Read the model definition and answer for the solid it produces. Units are mm, in the model's axes. A direction names the side the tool comes from. Round coordinates to 2 decimals unless told otherwise and drop trailing zeros. Loops run counter-clockwise (first coordinate to the right, second up) from the corner with the lowest first, then second, coordinate; pieces in that order, holes last. Notation, with made-up numbers: (-5.5, 29) -> (36.5, 29) arc R17 ccw to (36.5, 43) -> close; hole circle Ø5 at (-29.75, 14). An arc over 180 degrees is marked (long way). Put each result on its own line as item: value.
from build123d import *

# Parameters (mm, degrees)
SKETCH_1_W         = 5.2
SKETCH_1_H         = 5.2
EXTRUDE_1_DEPTH    = 0.8
CHAMFER_1_SIZE     = 1
EXTRUDE_1_2_DEPTH  = 0.4
SKETCH_2_R         = 1
EXTRUDE_1110_DEPTH = 1.1
SKETCH_4_W         = 0.6
SKETCH_4_H         = 2.66831223
EXTRUDE_2_DEPTH    = 0.2


with BuildPart() as part:
    # 草图1 → Extrude 1 (new body)
    with BuildSketch(Plane(origin=(0, 0, 0), x_dir=(1, 0, 0), z_dir=(0, 1, 0))):
        Rectangle(SKETCH_1_W, SKETCH_1_H)
    extrude(amount=EXTRUDE_1_DEPTH)

    # 倒角1
    chamfer_1_edges = [part.edges().sort_by_distance(p)[0] for p in [
        (-2.6, 0.4, -2.6),
        (2.6, 0.4, -2.6),
        (2.6, 0.4, 2.6),
        (-2.6, 0.4, 2.6),
    ]]
    chamfer(chamfer_1_edges, length=CHAMFER_1_SIZE)

    # 草图3 → Extrude 1 2 (add)
    with BuildSketch(Plane(origin=(0, 0.8, 0), x_dir=(1, 0, 0), z_dir=(0, 1, 0))):
        Polygon((-2.1, 1.392893219), (-2.1, -1.392893219), (-1.392893219, -2.1), (1.392893219, -2.1), (2.1, -1.392893219), (2.1, 1.392893219), (1.392893219, 2.1), (-1.392893219, 2.1), align=None)
    extrude(amount=EXTRUDE_1_2_DEPTH)

    # 草图2 → Extrude 1110 (add)
    with BuildSketch(Plane(origin=(0, 1.2, 0), x_dir=(-1, 0, 0), z_dir=(0, 1, 0))):
        with Locations(Location((0, 0, 0), (0, 0, 90))):
            Circle(SKETCH_2_R)
    extrude(amount=EXTRUDE_1110_DEPTH)

    # 草图4 → 凸台-拉伸2 (add)
    with BuildSketch(Plane.XZ):
        with Locations((-1.85, 2.465843885)):
            Rectangle(SKETCH_4_W, SKETCH_4_H)
        with Locations((1.85, 2.465843885)):
            Rectangle(SKETCH_4_W, SKETCH_4_H)
        with Locations((1.85, -2.465843885)):
            Rectangle(SKETCH_4_W, SKETCH_4_H)
        with Locations((-1.85, -2.465843885)):
            Rectangle(SKETCH_4_W, SKETCH_4_H)
    extrude(amount=-EXTRUDE_2_DEPTH)


solid = part.part
Item 1: Which of the six approach directions +Z, -Z, +X, -X, +Y, -Y give full straight-line access (tool end or side, diameter ignored) to faces 1 (the flat face through (0, 2.3, 0)), 2 (the cylindrical face through (-1, 2, 0))?
Derived:
face 1: +Z, -Z, +X, -X, +Y
face 2: +Y
Item 2: The part is cut by section B-B (x = 0). Determine the outline of the cut face in (y, z), then the cut area to 3 significant figures.
Derived:
outline: (0, -2.6) -> (0.8, -2.6) -> (0.8, -2.1) -> (1.2, -2.1) -> (1.2, -1) -> (2.3, -1) -> (2.3, 1) -> (1.2, 1) -> (1.2, 2.1) -> (0.8, 2.1) -> (0.8, 2.6) -> (0, 2.6) -> close
area: 8.04 mm^2
Item 3: Flat-ended cylindrical pins translate along their axes: pin 1 Ø1 at (y, z) = (2, -2.5) entering from -X; pin 2 Ø0.5 at (x, z) = (-2, -3) entering from +Y; pin 3 Ø1 at (y, z) = (1, -3) entering from -X; pin 4 Ø0.9 at (x, y) = (-0.5, 0.5) entering from +Z. Find the tip coordinate at first contact, or state that the pin passes through.
Derived:
pin 1: passes through
pin 2: stops at y = 0.2
pin 3: stops at x = -1.66
pin 4: stops at z = 2.6
Item 4: The part is cut by section C-C (y = 1.05). Determine the outline of the cut face in (x, z), then the cut area to 3 significant figures.
Derived:
outline: (-2.1, -1.39) -> (-1.39, -2.1) -> (1.39, -2.1) -> (2.1, -1.39) -> (2.1, 1.39) -> (1.39, 2.1) -> (-1.39, 2.1) -> (-2.1, 1.39) -> close
area: 16.6 mm^2
Item 5: Find the intervals of material crossed by line 1 along Y through (x, z) = (2, 1); line 2 along Y through (x, z) = (-0.75, 2.5); line 3 along X through (y, z) = (0.9, -1), in increasing order.
Derived:
line 1: y = 0 to 1.2
line 2: y = 0 to 0.8
line 3: x = -2.1 to 2.1
Item 6: The part is cut by section D-D (z = 2.5). Determine the outline of the cut face in (x, y), then the cut area to 3 significant figures.
Derived:
outline: (-2.15, 0) -> (2.15, 0) -> (2.15, 0.2) -> (1.7, 0.2) -> (1.7, 0.8) -> (-1.7, 0.8) -> (-1.7, 0.2) -> (-2.15, 0.2) -> close
area: 2.90 mm^2
Item 7: The part is cut by section A-A (z = -3). Determine the outline of the cut face in (x, y), then the cut area to 3 significant figures.
Derived:
outline: (-2.15, 0) -> (-1.55, 0) -> (-1.55, 0.2) -> (-2.15, 0.2) -> close; (1.55, 0) -> (2.15, 0) -> (2.15, 0.2) -> (1.55, 0.2) -> close
area: 0.240 mm^2
